Check sheet for the modelled part. Datum: model origin and axes. Units: mm. Round coordinates to 2 decimals unless told otherwise and drop trailing zeros. Order: outer loops, then holes, each group sorted by start corner. A loop starts at its lowest first (then second) coordinate and runs counter-clockwise, first axis right, second up. Notation, with made-up numbers: (49, -24) -> (72, -24) arc R20 cw to (72, -5) -> close; hole circle Ø9 at (35.5, -36). An arc over 180 degrees is marked (long way). Answer in a Markdown table with one row per item.
from build123d import *

# Parameters (mm, degrees)
BOSS_EXTRUDE1_DEPTH   = 1
SKETCH3_W             = 1
SKETCH3_H             = 3
BOSS_EXTRUDE2_DEPTH   = 5
F_1_5MM_DOWEL_HOLE1_D = 1.5


with BuildPart() as part:
    # Sketch1 → Boss-Extrude1 (new body)
    with BuildSketch(Plane.XY):
        with BuildLine():
            Line((1.776501472, 1.5), (0.276501472, 1.5))
            Line((0.276501472, 1.5), (0.276501472, -1.5))
            Line((0.276501472, -1.5), (1.776501472, -1.5))
            ThreePointArc((1.776501472, -1.5), (3.276501472, 0), (1.776501472, 1.5))
        make_face()
    extrude(amount=BOSS_EXTRUDE1_DEPTH)

    # Sketch3 → Boss-Extrude2 (add)
    with BuildSketch(Plane.ZY.offset(-0.276501472)):
        with Locations((0.5, 0)):
            Rectangle(SKETCH3_W, SKETCH3_H)
    extrude(amount=BOSS_EXTRUDE2_DEPTH)

    # Ø1.5mm Dowel Hole1 (through all)
    with Locations(Plane(origin=(0, 0, 0), x_dir=(-1, 0, 0), z_dir=(0, 0, -1))):
        with Locations((3.3, 0)):
            Hole(F_1_5MM_DOWEL_HOLE1_D / 2)

    # Sketch8 → CSK SLOT for M1.6 Countersunk Flat Head Screw1 (revolve, cut)
    with BuildSketch(Plane(origin=(1.776501472, 0, 1), x_dir=(0, -1, 0), z_dir=(1, 0, 0))):
        Polygon((0, 0), (0, 1), (0.9, 1), (0.9, 0.9), (1.8, 0), align=None)
    revolve(axis=Axis((1.776501472, 0, 7.35), (0, 0, -1)), mode=Mode.SUBTRACT)


solid = part.part
Item 1: Scan lines: line 1 (X direction, y = -0.1, z = 0.45); line 2 (Y direction, x = -3.3, z = 0.65); line 3 (X direction, y = 0.1, z = 0.25). Record each from-to range of solid material in increasing order. Write a range as [from, to].
Result sheet:
| item | result |
|---|---|
| line 1 | x = [-4.72, -4.04], [-2.56, 0.53], [3.02, 3.27] |
| line 2 | y = [-1.5, -0.75], [0.75, 1.5] |
| line 3 | x = [-4.72, -4.04], [-2.56, 0.73], [2.82, 3.27] |
Item 2: Cross-section at A-A (y = 0). Record the boundary of the cut face in (x, z).
Result sheet:
| item | result |
|---|---|
| outline | (-4.72, 0) -> (-4.05, 0) -> (-4.05, 1) -> (-4.72, 1) -> close; (-2.55, 0) -> (0.88, 0) -> (0.88, 0.1) -> (-0.02, 1) -> (-2.55, 1) -> close; (2.68, 0) -> (3.28, 0) -> (3.28, 0.7) -> (2.68, 0.1) -> close |
Item 3: Cross-section at D-D (y = 0.35). State how many separate pieces and enclosed holes the cut face has, and give its area (3 significant figures).
Result sheet:
| item | result |
|---|---|
| separate pieces | 3 |
| enclosed holes | 0 |
| area | 4.17 mm^2 |
Item 4: Mould release check, pull along Y, two halves, no side actions. Record for faces 1 (the flat face through (-4.723, 0, 0.5)), 2 (the cylindrical face through (3.276, -0.033, 0.345)), 3 (the flat face through (-1.4, -1.5, 0.5)), 4 (the cylindrical face through (-2.61, -0.29, 0.51)): pulls with the +Y half, pulls with the -Y half, needs draft (parallel to the pull), parting line crosses it, or undercut.
Result sheet:
| item | result |
|---|---|
| face 1 | needs draft |
| face 2 | parting line crosses it |
| face 3 | pulls with the -Y half |
| face 4 | undercut |
Item 5: Cross-section at B-B (x = -3.3). Record the boundary of the cut face in (y, z), and give its area (3 significant figures).
Result sheet:
| item | result |
|---|---|
| outline | (-1.5, 0) -> (-0.75, 0) -> (-0.75, 1) -> (-1.5, 1) -> close; (0.75, 0) -> (1.5, 0) -> (1.5, 1) -> (0.75, 1) -> close |
| area | 1.50 mm^2 |
Item 6: Cross-section at C-C (z = 0.35). Record the boundary of the cut face in (x, y), and give its area (3 significant figures).
Result sheet:
| item | result |
|---|---|
| outline | (-4.72, -1.5) -> (1.78, -1.5) arc R1.5 ccw to (1.78, 1.5) -> (-4.72, 1.5) -> close; hole circle Ø1.5 at (-3.3, 0); hole circle Ø2.3 at (1.78, 0) |
| area | 17.1 mm^2 |
